```python
from build123d import *

# Parameters (mm, degrees)
F0_R     = 7
F0_R_2   = 1.5
F1_DEPTH = 8.13
F2_R     = 2
F3_R     = 2


with BuildPart() as f1:
    # F0 (on Top) → F1 (new body)
    with BuildSketch(Plane.XY):
        Circle(F0_R)
        Circle(F0_R_2, mode=Mode.SUBTRACT)
    extrude(amount=F1_DEPTH)

    # F2
    f2_edges = [f1.edges().sort_by_distance(p)[0] for p in [
        (-7, 0, 8.13),
    ]]
    fillet(f2_edges, radius=F2_R)

    # F3
    f3_edges = [f1.edges().sort_by_distance(p)[0] for p in [
        (-7, 0, 0),
    ]]
    fillet(f3_edges, radius=F3_R)


solid = f1.part
```
Verification items for the finished model (mm, model axes). Round coordinates to 2 decimals unless told otherwise and drop trailing zeros. Write each loop counter-clockwise with the first axis right and the second up, starting at its lowest first coordinate (ties: lowest second). Pieces come first, ordered by that corner, then holes. Notation, with made-up numbers: (9.5, 87) - (26.5, 87) arc R20 cw to (26.5, 99) - close; hole circle Ø9 at (48.5, -24). An arc over 180 degrees is marked (long way). Answer as a JSON object with one key per item and string values. Group by question number.
Q1. Mould release check, pull along X, two halves, no side actions. Record for faces 1 (the cylindrical face through (-1.5, 0.07, 4.01)), 2 (the flat face through (-1.2, 1.2, 0)), 3 (the cylindrical face through (6.466, -2.681, 4.036)): released by +X, released by -X, zero draft, split by the parting line, or undercut.
Q2. Section check A-A, the plane y = 0. Enter the section's corners in (x, z).
Q3. Section check C-C, the plane z = 1.5. Enter the section's corners in (x, y).
Q4. Thickness scan on line 1 (Y direction, x = 0, z = 6); line 2 (Y direction, x = -0.75, z = 7.75); line 3 (Z direction, x = -5.25, y = -1.5). Record the ranges inside material, lowest first.
Q5. Section check D-D, the plane z = 0.5. Enter the section's corners in (x, y).
Q6. Go/stop test with flat-tipped pins: pin 1 Ø2.5 at (x, y) = (0, 0) entering from +Z; pin 2 Ø2 at (y, z) = (-2.5, 2.5) entering from -X; pin 3 Ø1 at (x, z) = (4, 4) entering from +Y; pin 4 Ø2 at (y, z) = (1.5, 4) entering from -X. Record where each tip stops, or that it passes through.
Found:
{
 "1": {"face 1": "undercut", "face 2": "zero draft", "face 3": "split by the parting line"},
 "2": {"outline": "(-7, 2) arc R2 ccw to (-5, 0) - (-1.5, 0) - (-1.5, 8.13) - (-5, 8.13) arc R2 ccw to (-7, 6.13) - close; (1.5, 0) - (5, 0) arc R2 ccw to (7, 2) - (7, 6.13) arc R2 ccw to (5, 8.13) - (1.5, 8.13) - close"},
 "3": {"outline": "circle Ø13.87 at (0, 0); hole circle Ø3 at (0, 0)"},
 "4": {"line 1": "y = -7 to -1.5, 1.5 to 7", "line 2": "y = -6.13 to -1.3, 1.3 to 6.13", "line 3": "z = 0.05 to 8.08"},
 "5": {"outline": "circle Ø12.65 at (0, 0); hole circle Ø3 at (0, 0)"},
 "6": {"pin 1": "passes through", "pin 2": "stops at x = -6.84", "pin 3": "stops at y = 6.06", "pin 4": "stops at x = -6.98"}
}
